Verification items for the finished model (mm, model axes). Face numbers are marked on the shaded views. A direction names the side the tool comes from. Round coordinates to 2 decimals unless told otherwise and drop trailing zeros. Order: outer loops, then holes, each group sorted by start corner. A loop starts at its lowest first (then second) coordinate and runs counter-clockwise, first axis right, second up. Notation, with made-up numbers: (6, -35) -> (40, -35) arc R33 ccw to (40, -3) -> close; hole circle Ø6 at (75, -5.5). An arc over 180 degrees is marked (long way). Answer in a Markdown table with one row per item. Add a question column.
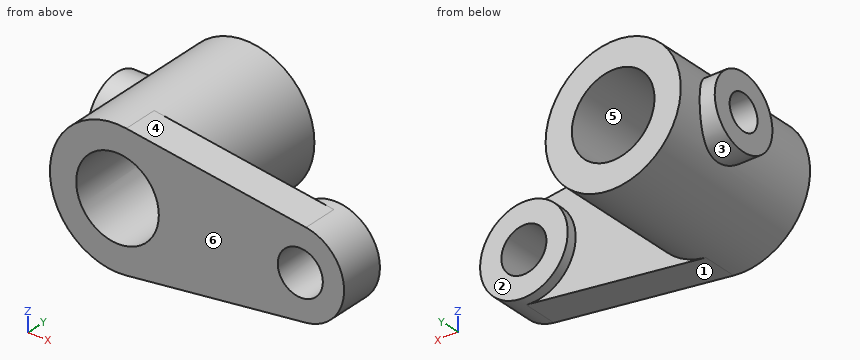
```python
from build123d import *

# Parameters (mm, degrees)
EXTRUDE_1_DEPTH     = 14
SKETCH_2_R          = 27
EXTRUDE_2_DEPTH     = 65
SKETCH_3_R          = 17.5
EXTRUDE_3_DEPTH     = 18
SKETCH_4_R          = 14.5
EXTRUDE_4_DEPTH     = 33
SKETCH_5_R          = 16.5
CUT_EXTRUDE_1_DEPTH = 66.0000001
SKETCH_6_R          = 9
CUT_EXTRUDE_2_DEPTH = 19.0000001
SKETCH_7_R          = 7
CUT_EXTRUDE_3_DEPTH = 33


with BuildPart() as part:
    # 草图1 → 凸台-拉伸1 (new body)
    with BuildSketch(Plane(origin=(0, 0, 0), x_dir=(1, 0, 0), z_dir=(0, 1, 0))):
        with BuildLine():
            Line((3.51369863, -26.770392637), (75.27739726, -17.351180413))
            ThreePointArc((75.27739726, -17.351180413), (90.5, 0), (75.27739726, 17.351180413))
            Line((75.27739726, 17.351180413), (3.51369863, 26.770392637))
            ThreePointArc((3.51369863, 26.770392637), (-27, 0), (3.51369863, -26.770392637))
        make_face()
    extrude(amount=EXTRUDE_1_DEPTH)

    # 草图2 → 凸台-拉伸2 (add)
    with BuildSketch(Plane(origin=(0, 0, 0), x_dir=(1, 0, 0), z_dir=(0, 1, 0))):
        Circle(SKETCH_2_R)
    extrude(amount=EXTRUDE_2_DEPTH)

    # 草图3 → 凸台-拉伸3 (add)
    with BuildSketch(Plane(origin=(0, 0, 0), x_dir=(1, 0, 0), z_dir=(0, 1, 0))):
        with Locations((73, 0)):
            Circle(SKETCH_3_R)
    extrude(amount=EXTRUDE_3_DEPTH)

    # 草图4 → 凸台-拉伸4 (add)
    with BuildSketch(Plane(origin=(0, 0, 0), x_dir=(0, 0, -1), z_dir=(1, 0, 0))):
        with Locations((0, 41)):
            Circle(SKETCH_4_R)
    extrude(amount=-EXTRUDE_4_DEPTH)

    # 草图5 → 切除-拉伸1 (cut, through all)
    with BuildSketch(Plane(origin=(0, 65, 0), x_dir=(1, 0, 0), z_dir=(0, 1, 0))):
        Circle(SKETCH_5_R)
    extrude(amount=-CUT_EXTRUDE_1_DEPTH, mode=Mode.SUBTRACT)

    # 草图6 → 切除-拉伸2 (cut, through all)
    with BuildSketch(Plane(origin=(0, 18, 0), x_dir=(1, 0, 0), z_dir=(0, 1, 0))):
        with Locations((73, 0)):
            Circle(SKETCH_6_R)
    extrude(amount=-CUT_EXTRUDE_2_DEPTH, mode=Mode.SUBTRACT)

    # 草图7 → 切除-拉伸3 (cut)
    with BuildSketch(Plane.ZY.offset(33)):
        with Locations((0, 41)):
            Circle(SKETCH_7_R)
    extrude(amount=-CUT_EXTRUDE_3_DEPTH, mode=Mode.SUBTRACT)


solid = part.part
```
1) Cross-section at C-C, the plane y = 41. Record the boundary of the cut face in (x, z).
2) Draft check along Z on the marked faces 4, 5 and 6. Enter one of: +Z half, -Z half, draft (parallel to the pull), parting line (faces both ways), or undercut.
3) Cross-section at D-D, the plane y = 50. Record the boundary of the cut face in (x, z).
4) Thickness scan on L1, parallel to X at y = 12, z = 0; L2, parallel to Z at x = 0, y = 21; L3, parallel to Y at x = 42.5, z = 18.5. Record the ranges inside material, lowest first. Write a range as [from, to].
5) Cross-section at B-B, the plane z = 0. Record the boundary of the cut face in (x, y).
6) Tool access check on the marked faces 1, 2 and 3. Record the directions out of +Z, -Z, +X, -X, +Y, -Y that give a thin tool (end or side, any length) a straight path to the whole face; none if there is none.
7) Depth check by flat-ended pin: P1, Ø12, axis at y = 54.5, z = 8, coming from the +X side; P2, Ø4, axis at x = -19.5, y = 11, coming from the +Z side; P3, Ø10, axis at x = 56, z = 9.5, coming from the +Y side; P4, Ø11, axis at x = 73, z = 0, coming from the -Y side. Enter the tip coordinate at first touch or a pass-through.
8) Cross-section at A-A, the plane x = 0. Record the boundary of the cut face in (y, z).
Results below:
| question | item | result |
|---|---|---|
| 1 | outline | (-33, -14.5) -> (-22.78, -14.5) arc R27 ccw (long way) to (-22.78, 14.5) -> (-33, 14.5) -> (-33, 7) -> (-14.94, 7) arc R16.5 cw (long way) to (-14.94, -7) -> (-33, -7) -> close |
| 2 | face 4 | +Z half |
| 2 | face 5 | undercut |
| 2 | face 6 | draft |
| 3 | outline | (-33, -11.37) -> (-24.49, -11.37) arc R27 ccw (long way) to (-24.49, 11.37) -> (-33, 11.37) -> close; hole circle Ø33 at (0, 0) |
| 4 | L1 | [-27, -16.5], [16.5, 64], [82, 90.5] |
| 4 | L2 | [-27, -16.5], [16.5, 27] |
| 4 | L3 | [0, 14] |
| 5 | outline | (-33, 26.5) -> (-27, 26.5) -> (-27, 0) -> (-16.5, 0) -> (-16.5, 34) -> (-33, 34) -> close; (-33, 48) -> (-16.5, 48) -> (-16.5, 65) -> (-27, 65) -> (-27, 55.5) -> (-33, 55.5) -> close; (16.5, 0) -> (64, 0) -> (64, 18) -> (55.5, 18) -> (55.5, 14) -> (27, 14) -> (27, 65) -> (16.5, 65) -> close; (82, 0) -> (90.5, 0) -> (90.5, 18) -> (82, 18) -> close |
| 6 | face 1 | -Z, +X, +Y, -Y |
| 6 | face 2 | +Z, -Z, +X, +Y |
| 6 | face 3 | -X |
| 7 | P1 | x = 26.93 |
| 7 | P2 | z = 20.56 |
| 7 | P3 | y = 18 |
| 7 | P4 | through |
| 8 | outline | (0, -27) -> (65, -27) -> (65, -16.5) -> (0, -16.5) -> close; (0, 16.5) -> (65, 16.5) -> (65, 27) -> (0, 27) -> close |
